from build123d import *

# Parameters (mm, degrees)
SKETCH1_R           = 2.5
BOSS_EXTRUDE1_DEPTH = 3
SKETCH2_R           = 5
CUT_EXTRUDE1_DEPTH  = 1.5


with BuildPart() as part:
    # Sketch1 → Boss-Extrude1 (new body)
    with BuildSketch(Plane.XY):
        Polygon((-57, 30), (57, 30), (72, 15), (72, -15), (57, -30), (-57, -30), (-72, -15), (-72, 15), align=None)
        with Locations((-61, 10)):
            Circle(SKETCH1_R, mode=Mode.SUBTRACT)
        with Locations(Location((61, 10, 0), (0, 0, 180))):
            Circle(SKETCH1_R, mode=Mode.SUBTRACT)
        with Locations((61, -10)):
            Circle(SKETCH1_R, mode=Mode.SUBTRACT)
        with Locations(Location((-61, -10, 0), (0, 0, 180))):
            Circle(SKETCH1_R, mode=Mode.SUBTRACT)
    extrude(amount=BOSS_EXTRUDE1_DEPTH)

    # Sketch2 → Cut-Extrude1 (cut)
    with BuildSketch(Plane.XY.offset(3)):
        with Locations((-61, -10)):
            Circle(SKETCH2_R)
        with Locations((-61, 10)):
            Circle(SKETCH2_R)
        with Locations((61, 10)):
            Circle(SKETCH2_R)
        with Locations((61, -10)):
            Circle(SKETCH2_R)
    extrude(amount=-CUT_EXTRUDE1_DEPTH, mode=Mode.SUBTRACT)


solid = part.part
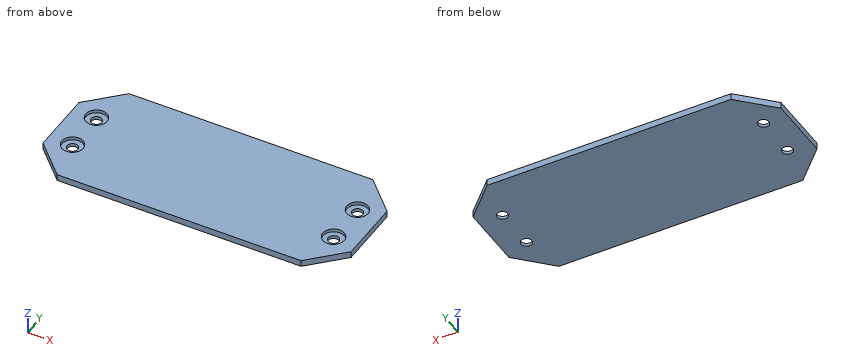
Check sheet for the modelled part. Datum: model origin and axes. Units: mm. Round coordinates to 2 decimals unless told otherwise and drop trailing zeros. Order: outer loops, then holes, each group sorted by start corner. A loop starts at its lowest first (then second) coordinate and runs counter-clockwise, first axis right, second up.
(1) Cross-section at A-A, the plane x = 61. Enter the section's corners in (y, z).
(2) Go/stop test with flat-tipped pins: P1, Ø6, axis at x = 61, y = 10, coming from the +Z side; P2, Ø4.5, axis at x = -61, y = 10, coming from the +Z side. Record where each tip stops, or that it passes through.
(3) Cross-section at C-C, the plane y = -25. Enter the section's corners in (x, z).
(4) Cross-section at B-B, the plane y = -10. Enter the section's corners in (x, z), and give its area (3 significant figures).
(5) Cross-section at D-D, the plane y = 21. Enter the section's corners in (x, z).
(6) Scan lines: probe 1 along X at (y, z) = (10, 1.15); probe 2 along Y at (x, z) = (-61, 1.2); probe 3 along X at (y, z) = (14, 2.35). Record each from-to range of solid material in increasing order.
Check sheet entries:
1. outline: (-26, 0) - (-12.5, 0) - (-12.5, 1.5) - (-15, 1.5) - (-15, 3) - (-26, 3) - close; (-7.5, 0) - (7.5, 0) - (7.5, 1.5) - (5, 1.5) - (5, 3) - (-5, 3) - (-5, 1.5) - (-7.5, 1.5) - close; (12.5, 0) - (26, 0) - (26, 3) - (15, 3) - (15, 1.5) - (12.5, 1.5) - close
2. P1: stops at z = 1.5
2. P2: passes through
3. outline: (-62, 0) - (62, 0) - (62, 3) - (-62, 3) - close
4. outline: (-72, 0) - (-63.5, 0) - (-63.5, 1.5) - (-66, 1.5) - (-66, 3) - (-72, 3) - close; (-58.5, 0) - (58.5, 0) - (58.5, 1.5) - (56, 1.5) - (56, 3) - (-56, 3) - (-56, 1.5) - (-58.5, 1.5) - close; (63.5, 0) - (72, 0) - (72, 3) - (66, 3) - (66, 1.5) - (63.5, 1.5) - close
4. area: 387 mm2
5. outline: (-66, 0) - (66, 0) - (66, 3) - (-66, 3) - close
6. probe 1: x = -72 to -63.5, -58.5 to 58.5, 63.5 to 72
6. probe 2: y = -26 to -12.5, -7.5 to 7.5, 12.5 to 26
6. probe 3: x = -72 to -64, -58 to 58, 64 to 72
